Read the model definition and answer for the solid it produces. Units are mm, in the model's axes. Face numbers are marked on the shaded views. Coordinates: 2 decimals unless noted, no trailing zeros. Order: outer loops, then holes, each group sorted by start corner. A loop starts at its lowest first (then second) coordinate and runs counter-clockwise, first axis right, second up. Notation, with made-up numbers: (17.25, 59.25) -> (62.25, 59.25) arc R23 ccw to (62.25, 73.25) -> close; hole circle Ø4 at (-7, 54). An arc over 180 degrees is marked (long way). Return JSON: item names as keys, results as strings. Group by question number.
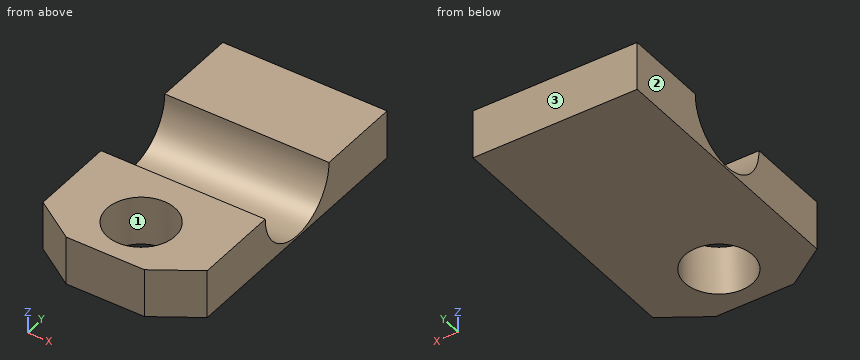
```python
from build123d import *

# Parameters (mm, degrees)
F0_W     = 192.6347911358
F0_H     = 216.3815796375
F1_DEPTH = 57.15
F2_R     = 39.8334565753
F3_DEPTH = 57.15
F5_D     = 109.22


with BuildPart() as f1:
    # F0 (on Top) → F1 (new body)
    with BuildSketch(Plane.XY):
        Rectangle(F0_W, F0_H)
    extrude(amount=-F1_DEPTH)

    # F2 (on face) → F3 (join)
    with BuildSketch(Plane.XY):
        Polygon((96.3173955679, -108.1907898188), (-96.3173955679, -108.1907898188), (-96.3173955679, -199.6307898188), (-46.5067504646, -232.6507898188), (45.1959193569, -232.6507898188), (96.3173955679, -199.6307898188), align=None)
        with Locations((0, -172.1784213857)):
            Circle(F2_R, mode=Mode.SUBTRACT)
    extrude(amount=-F3_DEPTH)

    # F5 (through all)
    with Locations(Plane(origin=(-96.3173955679, 0, 0), x_dir=(0, -1, 0), z_dir=(-1, 0, 0))):
        with Locations((45.72, 0)):
            Hole(F5_D / 2)


solid = f1.part
```
1. Find section B-B on x = 0. Determine the outline of the cut face in (y, z).
2. Find section C-C on y = -186. Determine the outline of the cut face in (x, z).
3. Find section A-A on z = -16.5. Determine the outline of the cut face in (x, y).
4. Find section D-D on z = -50. Determine the outline of the cut face in (x, y), and give its area (3 significant figures).
5. Straight lines are drawn through the part: L1, parallel to X at y = -173.5, z = -3; L2, parallel to Y at x = 0, z = -45; L3, parallel to Y at x = 0, z = -41. For each, find the intervals that lie inside material, in ascending order.
6. For a pull along Y with two mould halves and no side action, classify the marked faces 1, 2 and 3 as released by +Y, released by -Y, zero draft, split by the parting line, or undercut.
Result:
{
 "1": {"outline": "(-232.65, -57.15) -> (-212.01, -57.15) -> (-212.01, 0) -> (-232.65, 0) -> close; (-132.34, -57.15) -> (108.19, -57.15) -> (108.19, 0) -> (8.89, 0) arc R54.61 cw to (-100.33, 0) -> (-132.34, 0) -> close"},
 "2": {"outline": "(-96.32, -57.15) -> (-37.36, -57.15) -> (-37.36, 0) -> (-96.32, 0) -> close; (37.36, -57.15) -> (96.32, -57.15) -> (96.32, 0) -> (37.36, 0) -> close"},
 "3": {"outline": "(-96.32, -199.63) -> (-46.51, -232.65) -> (45.2, -232.65) -> (96.32, -199.63) -> (96.32, -97.78) -> (-96.32, -97.78) -> close; (-96.32, 6.34) -> (96.32, 6.34) -> (96.32, 108.19) -> (-96.32, 108.19) -> close; hole circle Ø79.67 at (0, -172.18)"},
 "4": {"outline": "(-96.32, -199.63) -> (-46.51, -232.65) -> (45.2, -232.65) -> (96.32, -199.63) -> (96.32, -67.68) -> (-96.32, -67.68) -> close; (-96.32, -23.76) -> (96.32, -23.76) -> (96.32, 108.19) -> (-96.32, 108.19) -> close; hole circle Ø79.67 at (0, -172.18)", "area": "50,500 mm^2"},
 "5": {"L1": "-96.32 to -39.81, 39.81 to 96.32", "L2": "-232.65 to -212.01, -132.34 to -76.66, -14.78 to 108.19", "L3": "-232.65 to -212.01, -132.34 to -81.79, -9.65 to 108.19"},
 "6": {"face 1": "undercut", "face 2": "zero draft", "face 3": "released by +Y"}
}
